from build123d import *

# Parameters (mm, degrees)
F0_W      = 25.4
F0_H      = 25.4
F0_R      = 1.5875
F1_DEPTH  = 25.4
F2_R      = 2.54
F3_DEPTH  = 7.62
F4_W      = 25.4
F4_H      = 12.7
F5_DEPTH  = 6.35
F6_W      = 6.35
F6_H      = 3.175
F7_DEPTH  = 12.7
F8_DEPTH  = 19.05
F9_R      = 1.5875
F10_DEPTH = 19.05


with BuildPart() as f1:
    # F0 (on Front) → F1 (new body)
    with BuildSketch(Plane.XZ):
        Rectangle(F0_W, F0_H)
        with Locations((-4.7625, 0)):
            Circle(F0_R, mode=Mode.SUBTRACT)
        with Locations((4.7625, 0)):
            Circle(F0_R, mode=Mode.SUBTRACT)
        with Locations((-4.7625, 0)):
            Circle(F0_R)
        with Locations((4.7625, 0)):
            Circle(F0_R)
    extrude(amount=-F1_DEPTH)

    # F2 (on face) → F3 (join)
    with BuildSketch(Plane(origin=(0, 25.4, 0), x_dir=(-1, 0, 0), z_dir=(0, 1, 0))):
        Circle(F2_R)
    extrude(amount=F3_DEPTH)

    # F4 (on face) → F5 (join)
    with BuildSketch(Plane(origin=(0, 33.02, 0), x_dir=(-1, 0, 0), z_dir=(0, 1, 0))):
        Rectangle(F4_W, F4_H)
    extrude(amount=F5_DEPTH)

    # F6 (on face) → F7 (join)
    with BuildSketch(Plane(origin=(0, 39.37, 0), x_dir=(-1, 0, 0), z_dir=(0, 1, 0))):
        with Locations((-9.525, 0)):
            Rectangle(F6_W, F6_H)
    extrude(amount=F7_DEPTH)

    # F0 (on Front) → F8 (cut)
    with BuildSketch(Plane.XZ):
        with Locations((-4.7625, 0)):
            Circle(F0_R)
        with Locations((4.7625, 0)):
            Circle(F0_R)
    extrude(amount=-F8_DEPTH, mode=Mode.SUBTRACT)

    # F9 (on face) → F10 (cut)
    with BuildSketch(Plane.YZ.offset(12.7)):
        with Locations((7.9375, 0)):
            Circle(F9_R)
        with Locations((17.4625, 0)):
            Circle(F9_R)
    extrude(amount=-F10_DEPTH, mode=Mode.SUBTRACT)


solid = f1.part
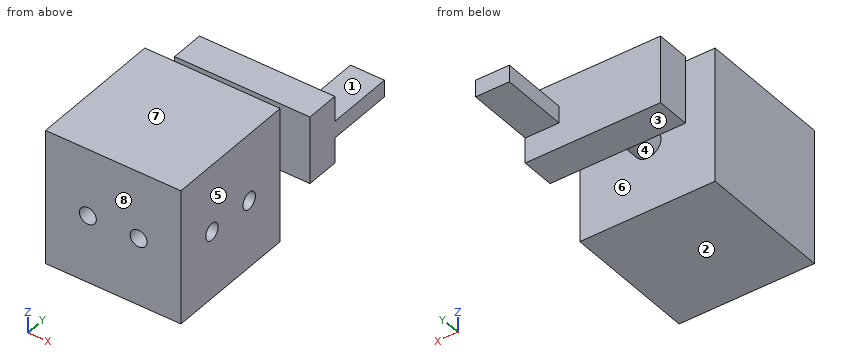
Can you work these out from the model? Positions are in its coordinate system, mm. Face numbers are marked on the shaded views. A direction names the side the tool comes from. Coordinates: 2 decimals unless noted, no trailing zeros. Write each loop counter-clockwise with the first axis right and the second up, starting at its lowest first coordinate (ties: lowest second). Pieces come first, ordered by that corner, then holes. Notation, with made-up numbers: (69, 57) - (116, 57) arc R6 cw to (116, 65) - close; hole circle Ø3 at (19.5, -33.75). An arc over 180 degrees is marked (long way). Return JSON: item names as keys, results as strings. Group by question number.
Item 1: If we section it at B-B (z = 5): Write out the boundary of the cut face in (x, y), then the cut area to 3 significant figures.
Item 2: I'm going to push flat-ended pins straight in: pin 1 Ø3 at (y, z) = (7.94, 0) entering from +X; pin 2 Ø1.6 at (y, z) = (44.5, 0.5) entering from -X; pin 3 Ø1.9 at (x, y) = (-4.5, 37.5) entering from +Z. Where does each tip first touch, or does it pass through?
Item 3: If we section it at D-D (y = 36.5): Write out the boundary of the cut face in (x, z), then the cut area to 3 significant figures.
Item 4: We'd pull the mould along Y, two halves only. Please class the marked faces 6, 7 and 8: pulls with the +Y half, pulls with the -Y half, needs draft (parallel to the pull), parting line crosses it, or undercut.
Item 5: Please list where these lines run through material, in increasing order: probe 1 along X at (y, z) = (12, 0) (3 decimals); probe 2 along Y at (x, z) = (-2.25, 0) (3 decimals); probe 3 along Y at (x, z) = (-5, 4.5).
Item 6: Which directions (+Z, -Z, +X, -X, +Y, -Y) give clear straight access to the entire face, cutting with the end or side of a thin tool? Please do the marked faces 1, 2, 3, 4 and 5.
Item 7: If we section it at A-A (x = 0): Count the separate pieces of the cut face and the enclosed holes in it, then the cut area to 3 significant figures.
Return value:
{
 "1": {"outline": "(-12.7, 0) - (12.7, 0) - (12.7, 25.4) - (-12.7, 25.4) - close; (-12.7, 33.02) - (12.7, 33.02) - (12.7, 39.37) - (-12.7, 39.37) - close", "area": "806 mm^2"},
 "2": {"pin 1": "stops at x = -6.35", "pin 2": "stops at x = 6.35", "pin 3": "stops at z = 6.35"},
 "3": {"outline": "(-12.7, -6.35) - (12.7, -6.35) - (12.7, 6.35) - (-12.7, 6.35) - close", "area": "323 mm^2"},
 "4": {"face 6": "undercut", "face 7": "needs draft", "face 8": "pulls with the -Y half"},
 "5": {"probe 1": "x = -12.7 to -6.35, -3.175 to 3.175, 6.35 to 12.7", "probe 2": "y = 0 to 6.35, 9.525 to 15.875, 19.05 to 39.37", "probe 3": "y = 0 to 25.4, 33.02 to 39.37"},
 "6": {"face 1": "+Z, +X, -X, +Y", "face 2": "-Z, +X, -X, +Y, -Y", "face 3": "-Z, +X, -X, +Y", "face 4": "none", "face 5": "+Z, -Z, +X, +Y, -Y"},
 "7": {"separate pieces": "1", "enclosed holes": "2", "area": "749 mm^2"}
}
